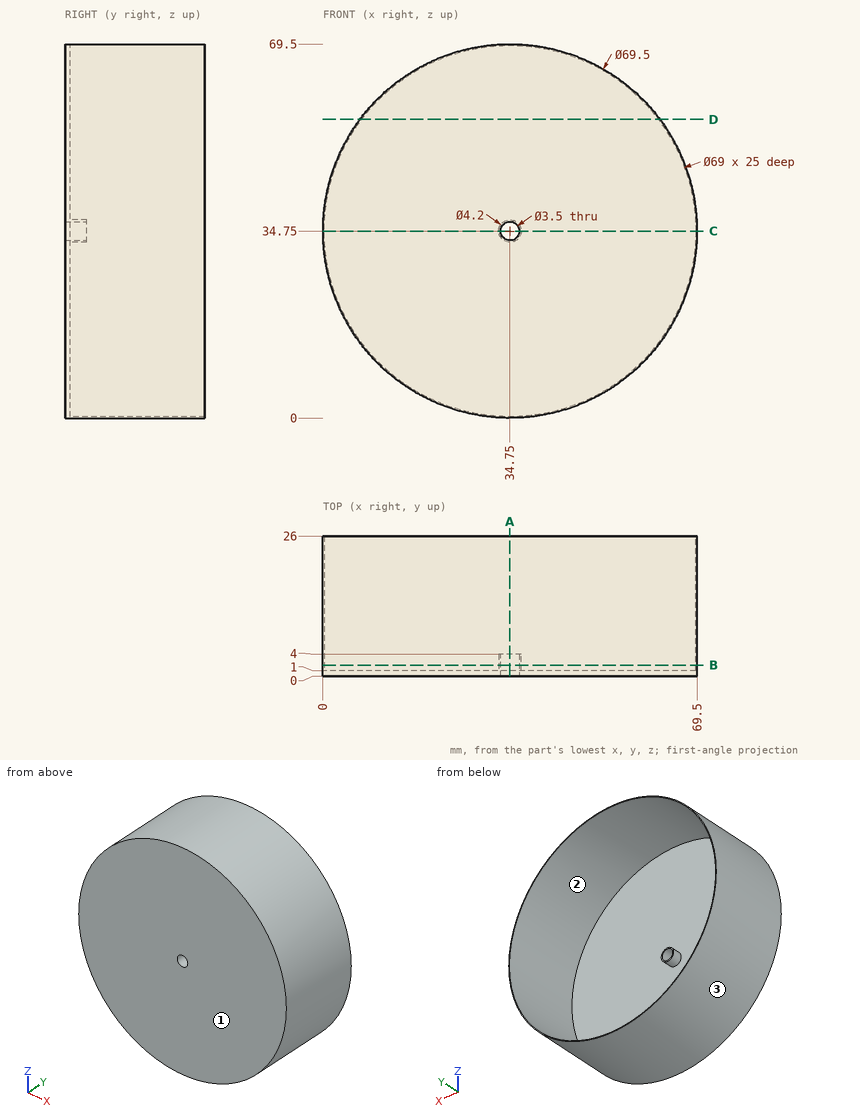
Drawing for the job (mm, zero at the part's lowest x, y, z). Round coordinates to 2 decimals unless told otherwise and drop trailing zeros. Loops run counter-clockwise (first coordinate to the right, second up) from the corner with the lowest first, then second, coordinate; pieces in that order, holes last. Notation, with made-up numbers: M 10,84 L 26,84 A9 ccw 26,96 Z; hole C 56,-0.5 d3. An arc over 180 degrees is marked long. Use a Markdown table: item, result. Add a question column.
(1) Flat gauge pins, fed straight in: pin 1 (4 mm diameter, centred on x = 34.75, z = 34.75, fed in from +Y); pin 2 (2 mm diameter, centred on x = 37, z = 26, fed in from +Y); pin 3 (5 mm diameter, centred on y = 13.5, z = 31.5, fed in from +X). Where does each tip first touch, or does it go through?
(2) Cut at C-C (z = 34.75). Give the cut face in (x, y).
(3) Cut at A-A (x = 34.75). Give the cut face in (y, z), and give its area (3 significant figures).
(4) Cut at D-D (z = 55.5). Give the cut face in (x, y), and give its area (3 significant figures).
(5) Drill centre lines: line 1 (Z direction, x = 34.75, y = 2.35); line 2 (Z direction, x = 34.75, y = 6.75). Where is each one in solid material? Low to high.
(6) Cut at B-B (y = 2). Give the cut face in (x, z), and give its area (3 significant figures).
(7) Pull direction X, two halves, no side cores. Call the marked faces 1, 2 and 3: +X half, -X half, draft (parallel to the pull), parting line (faces both ways), or undercut.
Geometry says:
| question | item | result |
|---|---|---|
| 1 | pin 1 | stops at y = 4 |
| 1 | pin 2 | stops at y = 1 |
| 1 | pin 3 | stops at x = 69.49 |
| 2 | outline | M 0,0 L 33,0 L 33,4 L 32.65,4 L 32.65,1 L 0.25,1 L 0.25,26 L 0,26 Z; M 36.5,0 L 69.5,0 L 69.5,26 L 69.25,26 L 69.25,1 L 36.85,1 L 36.85,4 L 36.5,4 Z |
| 3 | outline | M 0,0 L 26,0 L 26,0.25 L 1,0.25 L 1,32.65 L 4,32.65 L 4,33 L 0,33 Z; M 0,36.5 L 4,36.5 L 4,36.85 L 1,36.85 L 1,69.25 L 26,69.25 L 26,69.5 L 0,69.5 Z |
| 3 | area | 80.6 mm² |
| 4 | outline | M 6.88,0 L 62.62,0 L 62.62,26 L 62.31,26 L 62.31,1 L 7.19,1 L 7.19,26 L 6.88,26 Z |
| 4 | area | 71.4 mm² |
| 5 | line 1 | z = 0 to 0.25, 32.65 to 33, 36.5 to 36.85, 69.25 to 69.5 |
| 5 | line 2 | z = 0 to 0.25, 69.25 to 69.5 |
| 6 | outline | C 34.75,34.75 d69.5; C 34.75,34.75 d4.2; hole C 34.75,34.75 d69; hole C 34.75,34.75 d3.5 |
| 6 | area | 58.6 mm² |
| 7 | face 1 | draft |
| 7 | face 2 | undercut |
| 7 | face 3 | parting line |
